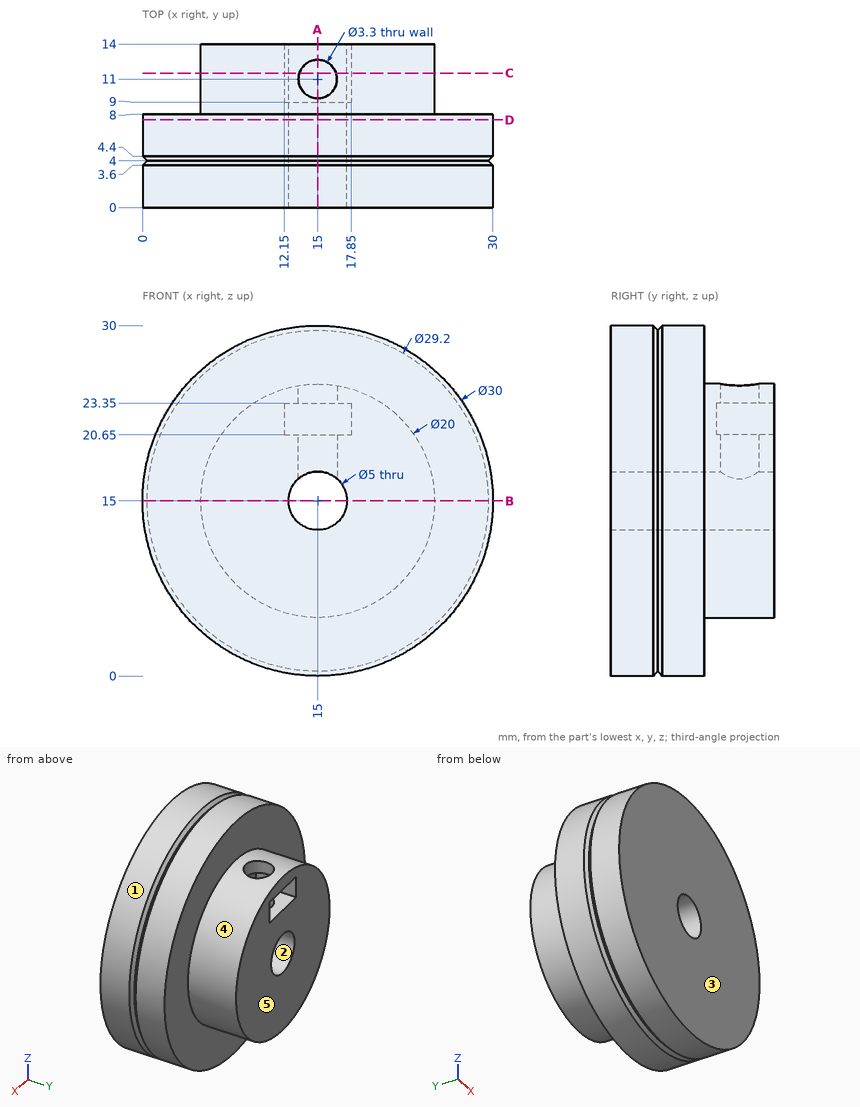
Source: three-view drawing plus pictorial views. Frame: mm from the lowest corner of the part. A direction names the side the tool comes from. Give positions to 0.01 mm unless a question says otherwise; leave off trailing zeros. Write each loop counter-clockwise with the first axis right and the second up, starting at its lowest first coordinate (ties: lowest second). Pieces come first, ordered by that corner, then holes. Notation, with made-up numbers: (70, 50.5) -> (108, 50.5) arc R6 ccw to (108, 61.5) -> close; hole circle Ø8 at (1, 39.5). An arc over 180 degrees is marked (long way). Answer in a Markdown table with one row per item.
(1) Pin query (flat end, axial travel): pin 1 (1.5 mm diameter, centred on x = 16, y = 11.5, fed in from +Z); pin 2 (4 mm diameter, centred on x = 15, y = 11, fed in from -Z); pin 3 (2 mm diameter, centred on y = 12, z = 22.5, fed in from +X). Return the tip coordinate at first contact, or that it passes through.
Answers below:
| item | result |
|---|---|
| pin 1 | z = 24.94 |
| pin 2 | z = 5 |
| pin 3 | x = 22.6 |
(2) Ray query, line 1 along Y through (x, z) = (15, 23.9); line 2 along Y through (x, z) = (4.75, 15.5); line 3 along X through (y, z) = (10.5, 15). Return the intervals inside material, ascending. Write a range as [from, to].
Answers below:
| item | result |
|---|---|
| line 1 | [0, 9.35], [12.65, 14] |
| line 2 | [0, 8] |
| line 3 | [5, 12.5], [17.5, 25] |
(3) Set-up query: the marked faces 4 and 5. Return all of +Z, -Z, +X, -X, +Y, -Y with unobstructed straight access to the full face (end or side cutting, diameter ignored); none if empty.
Answers below:
| item | result |
|---|---|
| face 4 | +Y |
| face 5 | +Z, -Z, +X, -X, +Y |
(4) Draft query along X for the marked faces 1, 2 and 3. Return one class per face: +X half, -X half, draft (parallel to the pull), parting line (faces both ways), or undercut.
Answers below:
| item | result |
|---|---|
| face 1 | parting line |
| face 2 | undercut |
| face 3 | draft |
(5) Section query D-D on y = 7.5. Return loops of the section in (x, z), then the cut area to 3 significant figures.
Answers below:
| item | result |
|---|---|
| outline | circle Ø30 at (15, 15); hole circle Ø5 at (15, 15) |
| area | 687 mm^2 |
(6) Section query C-C on y = 11.5. Return loops of the section in (x, z).
Answers below:
| item | result |
|---|---|
| outline | (12.15, 20.65) -> (12.15, 23.35) -> (13.43, 23.35) -> (13.43, 24.88) arc R10 ccw (long way) to (16.57, 24.88) -> (16.57, 23.35) -> (17.85, 23.35) -> (17.85, 20.65) -> (16.57, 20.65) -> (16.57, 16.94) arc R2.5 cw (long way) to (13.43, 16.94) -> (13.43, 20.65) -> close |
(7) Section query A-A on x = 15. State how many separate pieces and enclosed holes the cut face has, then the cut area to 3 significant figures.
Answers below:
| item | result |
|---|---|
| separate pieces | 4 |
| enclosed holes | 0 |
| area | 260 mm^2 |
(8) Section query B-B on z = 15. Return loops of the section in (x, y).
Answers below:
| item | result |
|---|---|
| outline | (0, 0) -> (12.5, 0) -> (12.5, 14) -> (5, 14) -> (5, 8) -> (0, 8) -> (0, 4.4) -> (0.4, 4) -> (0, 3.6) -> close; (17.5, 0) -> (30, 0) -> (30, 3.6) -> (29.6, 4) -> (30, 4.4) -> (30, 8) -> (25, 8) -> (25, 14) -> (17.5, 14) -> close |
